Work out the finished part from the listing and answer in its coordinate system (mm). A direction names the side the tool comes from. Coordinates: 2 decimals unless noted, no trailing zeros. Loops run counter-clockwise (first coordinate to the right, second up) from the corner with the lowest first, then second, coordinate; pieces in that order, holes last. Notation, with made-up numbers: (86, 81.25) - (121, 81.25) arc R15 cw to (121, 95.25) - close; hole circle Ø4 at (5.5, 25.5). An arc over 180 degrees is marked (long way). Write each question's results on one line, items separated by ' | '. Start each with the question number.
Item 1: Each of these flat-tipped pins is pushed along its axis until it touches: pin 1 Ø2 at (x, y) = (49.5, 61.5) entering from -Z; pin 2 Ø22 at (x, y) = (32.5, -3.5) entering from -Z; pin 3 Ø14.5 at (y, z) = (-58, 64.5) entering from +X; pin 4 Ø14.5 at (x, z) = (66, 178) entering from -Y. Where does it stop, or does it pass through?
Item 2: For a pull along Y with two mould halves and no side action, classify faces 1 (the face through (33, -211.161, 57)), 2 (the face through (58, -250.05, 183)), 3 (the face through (-1.63, -252.57, -13.4)), 4 (the face through (21, -254.05, 77)) as +Y half, -Y half, draft (parallel to the pull), parting line (faces both ways), or undercut.
Item 3: Consider probe 1 along X at (y, z) = (-253.05, 0); probe 2 along Z at (x, y) = (68, -251); probe 3 along Y at (x, z) = (38, 65). Determine where each line is inside the solid, lowest interval first. Write a range as [from, to].
Item 4: Section B-B, the plane x = 54.5 is taken. Write down the section's boundary in (y, z).
Item 5: Section A-A, the plane y = 127.5 is taken. Write down the section's boundary in (x, z), plus the area to 3 significant figures.
Item 6: A tool of negligible diameter and unlimited length cuts with its end or side. For faces 5 (the face through (22.5, 67, 98)), 6 (the face through (33, -137, 160.836)), 7 (the face through (29, -60, 197.3)), from which of +Z, -Z, +X, -X, +Y, -Y can it reach the whole face along a straight path? Write none if from no direction.
Item 7: Section C-C, the plane x = -100 is taken. Write down the section's boundary in (y, z).
from build123d import *

# Parameters (mm, degrees)
F0_R      = 6.5
F1_DEPTH  = 254.05
F2_W      = 502.1
F2_H      = 100
F3_DEPTH  = 140
F4_R      = 10
F5_W      = 508.1
F5_H      = 200
F6_DEPTH  = 4
F7_W      = 150
F7_H      = 160
F8_DEPTH  = 25
F9_W      = 190
F9_H      = 200
F10_DEPTH = 5
F11_W     = 170
F11_H     = 180
F12_DEPTH = 25
F13_W     = 318.1
F13_H     = 200
F14_DEPTH = 25
F16_DEPTH = 20
F17_R     = 6.5
F18_DEPTH = 318
F19_W     = 52
F19_H     = 310
F20_DEPTH = 30


with BuildPart() as f1:
    # F0 (on Front) → F1 (new body, symmetric)
    with BuildSketch(Plane.XZ):
        with BuildLine():
            Line((-13.5, 15), (-13.5, 0))
            ThreePointArc((-13.5, 0), (-1.3568709871, -13.4316380656), (13.227244611, -2.7))
            Line((13.227244611, -2.7), (13.5, -2.7))
            Line((13.5, -2.7), (13.5, 15))
            Line((13.5, 15), (13.5, 35))
            Line((13.5, 35), (-113.5, 35))
            Line((-113.5, 35), (-113.5, 15))
            Line((-113.5, 15), (-13.5, 15))
        make_face()
        Circle(F0_R, mode=Mode.SUBTRACT)
    extrude(amount=F1_DEPTH, both=True)

    # F2 (on face) → F3 (cut)
    with BuildSketch(Plane.YZ.offset(13.5)):
        Rectangle(F2_W, F2_H)
    extrude(amount=-F3_DEPTH, mode=Mode.SUBTRACT)

    # F4
    f4_edges = [f1.edges().sort_by_distance(p)[0] for p in [
        (-13.5, -252.55, 15),
        (-13.5, 252.55, 15),
    ]]
    fillet(f4_edges, radius=F4_R)

    # F5 (on face) → F6 (join)
    with BuildSketch(Plane.YZ.offset(13.5)):
        with Locations((0, 97.3)):
            Rectangle(F5_W, F5_H)
    extrude(amount=F6_DEPTH)

    # F7 (on face) → F8 (cut)
    with BuildSketch(Plane.YZ.offset(17.5)):
        with Locations((159.05, 97.3)):
            Rectangle(F7_W, F7_H)
    extrude(amount=-F8_DEPTH, mode=Mode.SUBTRACT)

    # F9 (on face) → F10 (join)
    with BuildSketch(Plane.YZ.offset(17.5)):
        with Locations((159.05, 97.3)):
            Rectangle(F9_W, F9_H)
    extrude(amount=F10_DEPTH)

    # F11 (on face) → F12 (cut)
    with BuildSketch(Plane.YZ.offset(17.5)):
        with Locations((159.05, 97.3)):
            Rectangle(F11_W, F11_H)
    extrude(amount=F12_DEPTH, mode=Mode.SUBTRACT)

    # F13 (on face) → F14 (join)
    with BuildSketch(Plane.YZ.offset(17.5)):
        with Locations((-95, 97.3)):
            Rectangle(F13_W, F13_H)
    extrude(amount=F14_DEPTH)

    # F15 (on face) → F16 (cut)
    with BuildSketch(Plane.YZ.offset(42.5)):
        with BuildLine():
            Line((-42.7234955132, 160.8355042394), (-234.0602389828, 160.8355042394))
            add(Edge.make_bspline(
                [(-234.0602389828, 160.8355042394), (-217.1074327426, 151.3089947091), (-196.7785844767, 119.4842501759), (-119.2925410931, 121.4843631106), (-84.3255399594, 123.5550247597)],
                knots=[0, 0, 0, 0, 0.4134970992, 1, 1, 1, 1], degree=3))
            ThreePointArc((-84.3255399594, 123.5550247597), (-80.0809052846, 134.4004465368), (-69.1307716391, 138.367141659))
            add(Edge.make_bspline(
                [(-69.1307716391, 138.367141659), (-47.0103981225, 137.0126396602), (1.6618247246, 135.6066305681), (26.4505103488, 126.2112086953), (41.4993381181, 122.1753671593)],
                knots=[0, 0, 0, 0, 0.5598213266, 1, 1, 1, 1], degree=3))
            ThreePointArc((41.4993381181, 122.1753671593), (51.4208114186, 140.9997574198), (41.4993381181, 159.8241476803))
            add(Edge.make_bspline(
                [(-42.7234955132, 160.8355042394), (-27.0416883232, 160.9222176304), (-1.4651588493, 161.1197494684), (29.1631212378, 160.1908804879), (41.4993381181, 159.8241476803)],
                knots=[0, 0, 0, 0, 0.5035967712, 1, 1, 1, 1], degree=3))
        make_face()
        with BuildLine():
            Line((21.5523498238, 73.3963885321), (-67.0575042699, 73.3963885321))
            add(Edge.make_bspline(
                [(-67.0575042699, 73.3963885321), (-85.0711185917, 100.9948365173), (-120.0462196172, 82.577282884), (-155.0213206427, 64.1597292506), (-120.7750741023, 45.1092301127), (-86.5288275619, 26.0587309749), (-67.4480830546, 53.317995912)],
                knots=[0.4207699255, 0.4207699255, 0.4207699255, 2.2257610437, 2.2257610437, 4.0307521619, 4.0307521619, 5.83574328, 5.83574328, 5.83574328], degree=2, weights=[1, 0.6196531961, 1, 0.6196531961, 1, 0.6196531961, 1]))
            Line((-67.4480830546, 53.317995912), (21.1617710391, 53.317995912))
            ThreePointArc((21.1617710391, 53.317995912), (31.2028666218, 63.1656647881), (21.5523498238, 73.3963885321))
        make_face()
        with BuildLine():
            ThreePointArc((-211.1607789993, 27.7673769742), (-200.8758932352, 17.4824912101), (-190.5910074711, 27.7673769742))
            Line((-190.5910074711, 27.7673769742), (-190.5910074711, 78.6157455295))
            Line((-190.5910074711, 78.6157455295), (-190.5910074711, 95.1955616474))
            Line((-190.5910074711, 95.1955616474), (-202.446475625, 119.7409853339))
            ThreePointArc((-202.446475625, 119.7409853339), (-208.6635845365, 122.1287897822), (-211.4351242781, 116.0729974508))
            add(Edge.make_bspline(
                [(-206.3090205193, 78.6157455295), (-203.2636096895, 79.3219361096), (-193.8499770894, 81.5048332746), (-204.3392460287, 102.1242097799), (-211.4351242781, 116.0729974508)],
                knots=[0, 0, 0, 0, 0.3235106955, 1, 1, 1, 1], degree=3))
            add(Edge.make_bspline(
                [(-211.1607789993, 84.4994708896), (-209.9125958931, 84.8049572899), (-206.9667390663, 85.5259406083), (-206.5494822717, 81.1421112915), (-206.3090205193, 78.6157455295)],
                knots=[0, 0, 0, 0, 0.4237080006, 1, 1, 1, 1], degree=3))
            Line((-211.1607789993, 84.4994708896), (-211.1607789993, 78.6157455295))
            Line((-211.1607789993, 78.6157455295), (-211.1607789993, 27.7673769742))
        make_face()
    extrude(amount=-F16_DEPTH, mode=Mode.SUBTRACT)

    # F17 (on face) → F18 (join)
    with BuildSketch(Plane.XZ.offset(254.05)):
        with BuildLine():
            Line((68.5, 197.3), (42.5, 197.3))
            Line((42.5, 197.3), (42.5, 168.3))
            Line((42.5, 168.3), (68.5, 168.3))
            ThreePointArc((68.5, 168.3), (83, 182.8), (68.5, 197.3))
        make_face()
        with Locations((68.5, 182.8)):
            Circle(F17_R, mode=Mode.SUBTRACT)
    extrude(amount=-F18_DEPTH)

    # F19 (on face) → F20 (cut)
    with BuildSketch(Plane.XY.offset(197.3)):
        with Locations((68.5, -95.05)):
            Rectangle(F19_W, F19_H)
    extrude(amount=-F20_DEPTH, mode=Mode.SUBTRACT)


solid = f1.part
Answer key:
1) pin 1: stops at z = 168.3 | pin 2: stops at z = -2.7 | pin 3: stops at x = 22.5 | pin 4: stops at y = -254.05
2) face 1: undercut | face 2: undercut | face 3: draft | face 4: -Y half
3) probe 1: x = [-13.5, -6.5], [6.5, 42.5] | probe 2: z = [168.3, 176.32], [189.28, 197.3] | probe 3: y = [-254.05, -211.16], [-190.59, -133.6], [31.07, 64.05]
4) outline: (-254.05, 168.3) - (-250.05, 168.3) - (-250.05, 197.3) - (-254.05, 197.3) - close; (59.95, 168.3) - (63.95, 168.3) - (63.95, 197.3) - (59.95, 197.3) - close
5) outline: (13.5, -2.7) - (22.5, -2.7) - (22.5, 7.3) - (17.5, 7.3) - (17.5, 17.3) - (13.5, 17.3) - close; (13.5, 177.3) - (17.5, 177.3) - (17.5, 187.3) - (22.5, 187.3) - (22.5, 197.3) - (13.5, 197.3) - close | area: 260 mm^2
6) face 5: +Z, -Z, +X, +Y | face 6: +X | face 7: +Z, +X, -X, +Y, -Y
7) outline: (-254.05, 15) - (-251.05, 15) - (-251.05, 35) - (-254.05, 35) - close; (251.05, 15) - (254.05, 15) - (254.05, 35) - (251.05, 35) - close
